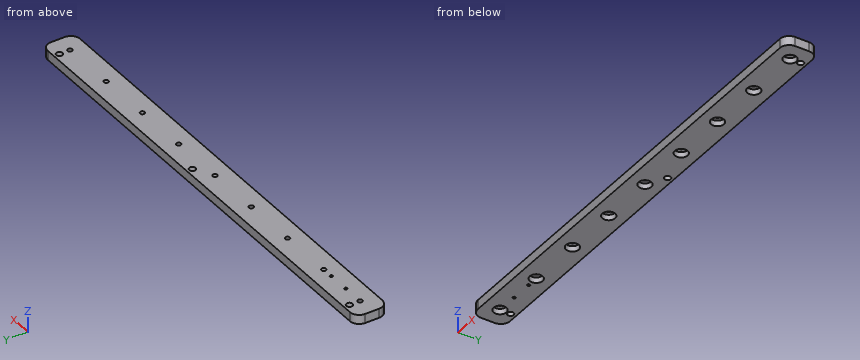
from build123d import *

# Parameters (mm, degrees)
ESQUISSE1_R             = 7
BOSS_EXTRU_1_DEPTH      = 10
BOSS_EXTRU_2_START      = -4
ESQUISSE2_R             = 7
ESQUISSE2_R_2           = 2.5
BOSS_EXTRU_2_DEPTH      = 4
ESQUISSE3_R             = 3.375
ENL_V_MAT_EXTRU_1_DEPTH = 261.780079761
ESQUISSE4_R             = 3.375
ENL_V_MAT_EXTRU_2_DEPTH = 261.780079761
ESQUISSE5_R             = 1.5
ENL_V_MAT_EXTRU_3_DEPTH = 261.780079761


with BuildPart() as part:
    # Esquisse1 → Boss.-Extru.1 (new body)
    with BuildSketch(Plane.XY):
        with BuildLine():
            Line((-250, 17.5), (250, 17.5))
            ThreePointArc((250, 17.5), (257.071067812, 14.571067812), (260, 7.5))
            Line((260, 7.5), (260, -7.5))
            ThreePointArc((260, -7.5), (257.071067812, -14.571067812), (250, -17.5))
            Line((250, -17.5), (-250, -17.5))
            ThreePointArc((-250, -17.5), (-257.071067812, -14.571067812), (-260, -7.5))
            Line((-260, -7.5), (-260, 7.5))
            ThreePointArc((-260, 7.5), (-257.071067812, 14.571067812), (-250, 17.5))
        make_face()
        with Locations((-240, 0)):
            Circle(ESQUISSE1_R, mode=Mode.SUBTRACT)
        with Locations((-180, 0)):
            Circle(ESQUISSE1_R, mode=Mode.SUBTRACT)
        with Locations((-120, 0)):
            Circle(ESQUISSE1_R, mode=Mode.SUBTRACT)
        with Locations((-60, 0)):
            Circle(ESQUISSE1_R, mode=Mode.SUBTRACT)
        Circle(ESQUISSE1_R, mode=Mode.SUBTRACT)
        with Locations((60, 0)):
            Circle(ESQUISSE1_R, mode=Mode.SUBTRACT)
        with Locations((120, 0)):
            Circle(ESQUISSE1_R, mode=Mode.SUBTRACT)
        with Locations((180, 0)):
            Circle(ESQUISSE1_R, mode=Mode.SUBTRACT)
        with Locations((240, 0)):
            Circle(ESQUISSE1_R, mode=Mode.SUBTRACT)
    extrude(amount=BOSS_EXTRU_1_DEPTH)

    # Esquisse2 → Boss.-Extru.2 (add)
    # profile 1 of 9: a face of its own
    with BuildSketch(Plane.XY.offset(10).offset(BOSS_EXTRU_2_START)):
        with Locations((-240, 0)):
            Circle(ESQUISSE2_R)
        with Locations((-240, 0)):
            Circle(ESQUISSE2_R_2, mode=Mode.SUBTRACT)
    # profile 2 of 9: a face of its own
    with BuildSketch(Plane.XY.offset(10).offset(BOSS_EXTRU_2_START)):
        with Locations((-180, 0)):
            Circle(ESQUISSE2_R)
        with Locations((-180, 0)):
            Circle(ESQUISSE2_R_2, mode=Mode.SUBTRACT)
    # profile 3 of 9: a face of its own
    with BuildSketch(Plane.XY.offset(10).offset(BOSS_EXTRU_2_START)):
        with Locations((-120, 0)):
            Circle(ESQUISSE2_R)
        with Locations((-120, 0)):
            Circle(ESQUISSE2_R_2, mode=Mode.SUBTRACT)
    # profile 4 of 9: a face of its own
    with BuildSketch(Plane.XY.offset(10).offset(BOSS_EXTRU_2_START)):
        with Locations((-60, 0)):
            Circle(ESQUISSE2_R)
        with Locations((-60, 0)):
            Circle(ESQUISSE2_R_2, mode=Mode.SUBTRACT)
    # profile 5 of 9: a face of its own
    with BuildSketch(Plane.XY.offset(10).offset(BOSS_EXTRU_2_START)):
        Circle(ESQUISSE2_R)
        Circle(ESQUISSE2_R_2, mode=Mode.SUBTRACT)
    # profile 6 of 9: a face of its own
    with BuildSketch(Plane.XY.offset(10).offset(BOSS_EXTRU_2_START)):
        with Locations((60, 0)):
            Circle(ESQUISSE2_R)
        with Locations((60, 0)):
            Circle(ESQUISSE2_R_2, mode=Mode.SUBTRACT)
    # profile 7 of 9: a face of its own
    with BuildSketch(Plane.XY.offset(10).offset(BOSS_EXTRU_2_START)):
        with Locations((120, 0)):
            Circle(ESQUISSE2_R)
        with Locations((120, 0)):
            Circle(ESQUISSE2_R_2, mode=Mode.SUBTRACT)
    # profile 8 of 9: a face of its own
    with BuildSketch(Plane.XY.offset(10).offset(BOSS_EXTRU_2_START)):
        with Locations((180, 0)):
            Circle(ESQUISSE2_R)
        with Locations((180, 0)):
            Circle(ESQUISSE2_R_2, mode=Mode.SUBTRACT)
    # profile 9 of 9: a face of its own
    with BuildSketch(Plane.XY.offset(10).offset(BOSS_EXTRU_2_START)):
        with Locations((240, 0)):
            Circle(ESQUISSE2_R)
        with Locations((240, 0)):
            Circle(ESQUISSE2_R_2, mode=Mode.SUBTRACT)
    extrude(amount=BOSS_EXTRU_2_DEPTH)

    # Esquisse3 → Enlèv. mat.-Extru.1 (cut, through all)
    with BuildSketch(Plane.XY.offset(10)):
        with Locations((20.000000156, 11.500000313)):
            Circle(ESQUISSE3_R)
        with Locations((-239.999999844, 11.500000313)):
            Circle(ESQUISSE3_R)
    extrude(amount=-ENL_V_MAT_EXTRU_1_DEPTH, mode=Mode.SUBTRACT)

    # Esquisse4 → Enlèv. mat.-Extru.2 (cut, through all)
    with BuildSketch(Plane.XY.offset(10)):
        with Locations((240.000000156, 11.500000313)):
            Circle(ESQUISSE4_R)
    extrude(amount=-ENL_V_MAT_EXTRU_2_DEPTH, mode=Mode.SUBTRACT)

    # Esquisse5 → Enlèv. mat.-Extru.3 (cut, through all)
    with BuildSketch(Plane.XY.offset(10)):
        with Locations((-192.499999844, 0)):
            Circle(ESQUISSE5_R)
        with Locations((-216.499999844, 0)):
            Circle(ESQUISSE5_R)
    extrude(amount=-ENL_V_MAT_EXTRU_3_DEPTH, mode=Mode.SUBTRACT)


solid = part.part
Check sheet for the modelled part. Datum: model origin and axes. Units: mm. Give positions to 0.01 mm unless a question says otherwise; leave off trailing zeros. Use a Markdown table: item, result. Add a question column.
Q1. Go/stop test with flat-tipped pins: pin 1 (16 mm diameter, centred on x = 120, y = 0, fed in from +Z); pin 2 (4.5 mm diameter, centred on x = -180, y = 0, fed in from +Z); pin 3 (6.5 mm diameter, centred on x = 0, y = 0, fed in from -Z). Record where each tip stops, or that it passes through.
Q2. Sectioned sample at A-A, the plane z = 2. Give the number of separate pieces and of enclosed holes in the cut face, then the cut area to 3 significant figures.
Q3. Scan lines: line 1 along Y through (x, z) = (240, 3.85) (3 decimals); line 2 along Y through (x, z) = (240, 8.3) (3 decimals); line 3 along Y through (x, z) = (-60, 7.5). Record each from-to range of solid material in increasing order. Write a range as [from, to].
Verdict:
| question | item | result |
|---|---|---|
| 1 | pin 1 | z = 10 |
| 1 | pin 2 | through |
| 1 | pin 3 | z = 6 |
| 2 | separate pieces | 1 |
| 2 | enclosed holes | 14 |
| 2 | area | 16,600 mm^2 |
| 3 | line 1 | [-17.5, -7], [7, 8.125], [14.875, 17.5] |
| 3 | line 2 | [-17.5, -2.5], [2.5, 8.125], [14.875, 17.5] |
| 3 | line 3 | [-17.5, -2.5], [2.5, 17.5] |
